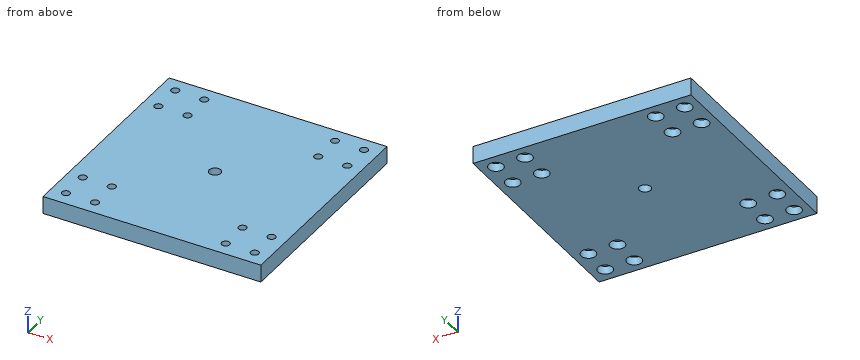
```python
from build123d import *

# Parameters (mm, degrees)
SKETCH1_W                                           = 150
SKETCH1_H                                           = 150
BOSS_EXTRUDE1_DEPTH                                 = 12
F_3_8_16_TAPPED_HOLE1_D                             = 7.9375
CBORE_FOR_M5_HEX_SOCKET_HEAD_CAP_SCREW1_D           = 5.5
CBORE_FOR_M5_HEX_SOCKET_HEAD_CAP_SCREW1_CBORE_D     = 10
CBORE_FOR_M5_HEX_SOCKET_HEAD_CAP_SCREW1_CBORE_DEPTH = 5.5


with BuildPart() as part:
    # Sketch1 → Boss-Extrude1 (new body)
    with BuildSketch(Plane.XY):
        Rectangle(SKETCH1_W, SKETCH1_H)
    extrude(amount=BOSS_EXTRUDE1_DEPTH)

    # 3/8-16 Tapped Hole1 (through all)
    with Locations(Plane.XY.offset(12)):
        with Locations((0, 0)):
            Hole(F_3_8_16_TAPPED_HOLE1_D / 2)

    # CBORE for M5 Hex Socket Head Cap Screw1 (through all)
    with Locations(Plane(origin=(0, 0, 0), x_dir=(1, 0, 0), z_dir=(0, 0, -1))):
        with Locations((-65, -65), (-45, -65), (-65, -45), (-65, 45), (-45, 65), (-65, 65), (65, 45), (65, 65), (45, 65), (45, -65), (65, -65), (65, -45), (-45, -45), (45, -45), (45, 45), (-45, 45)):
            CounterBoreHole(CBORE_FOR_M5_HEX_SOCKET_HEAD_CAP_SCREW1_D / 2, CBORE_FOR_M5_HEX_SOCKET_HEAD_CAP_SCREW1_CBORE_D / 2, CBORE_FOR_M5_HEX_SOCKET_HEAD_CAP_SCREW1_CBORE_DEPTH)


solid = part.part
```
Input: part model. Units: mm. Frame: model coordinates. Coordinates: 2 decimals unless noted, no trailing zeros. Loops run counter-clockwise (first coordinate to the right, second up) from the corner with the lowest first, then second, coordinate; pieces in that order, holes last. Notation, with made-up numbers: M -3.5,70.25 L 12.5,70.25 A17 ccw 12.5,75.25 Z; hole C -17.75,0.25 d5. An arc over 180 degrees is marked long. Use a Markdown table: item, result. Add a question column.
1) Section A-A, the plane z = 2.75. Give the number of separate pieces and of enclosed holes in the cut face, plus the area to 3 significant figures.
2) Section B-B, the plane x = 0. Return the cut outline in (y, z), plus the area to 3 significant figures.
3) Pin query (flat end, axial travel): P1, Ø5, axis at x = -64, y = 46.5, coming from the -Z side. Return the tip coordinate at first contact, or that it passes through.
4) Line query: L1, parallel to X at y = 45, z = 1.1; L2, parallel to Y at x = 45, z = 7.25. Output: solid intervals per line, ascending. Write a range as from..to.
Answer below:
| question | item | result |
|---|---|---|
| 1 | separate pieces | 1 |
| 1 | enclosed holes | 17 |
| 1 | area | 21,200 mm2 |
| 2 | outline | M -75,0 L -3.97,0 L -3.97,12 L -75,12 Z; M 3.97,0 L 75,0 L 75,12 L 3.97,12 Z |
| 2 | area | 1,700 mm2 |
| 3 | P1 | z = 5.5 |
| 4 | L1 | -75..-70, -60..-50, -40..40, 50..60, 70..75 |
| 4 | L2 | -75..-67.75, -62.25..-47.75, -42.25..42.25, 47.75..62.25, 67.75..75 |
